from build123d import *

# Parameters (mm, degrees)
SKETCH1_R                      = 4.25
BOSS_EXTRUDE1_DEPTH            = 10
BOSS_EXTRUDE2_START            = -5
BOSS_EXTRUDE2_DEPTH            = 15
SKETCH3_W                      = 175
SKETCH3_H                      = 10
BOSS_EXTRUDE3_DEPTH            = 51.25
SKETCH4_W                      = 160
SKETCH4_H                      = 117.5
CUT_EXTRUDE1_DEPTH             = 10
CUT_EXTRUDE1_DIRECTION_2_REACH = 219.644
SKETCH5_W                      = 175
SKETCH5_H                      = 117.5
CUT_EXTRUDE2_DEPTH             = 15
SKETCH6_W                      = 5
SKETCH6_H                      = 15
BOSS_EXTRUDE4_DEPTH            = 3
CUT_EXTRUDE3_REACH             = 222.327
SKETCH7_W                      = 145
SKETCH7_H                      = 12.5


with BuildPart() as part:
    # Sketch1 → Boss-Extrude1 (new body)
    with BuildSketch(Plane(origin=(0, 0, 0), x_dir=(1, 0, 0), z_dir=(0, 1, 0))):
        Polygon((-87.5, 6.25), (87.5, 6.25), (87.5, -17), (75, -17), (75, -6.25), (-75, -6.25), (-75, -17), (-87.5, -17), align=None)
        with Locations(Location((-80, 0, 0), (0, 0, 270))):
            Circle(SKETCH1_R, mode=Mode.SUBTRACT)
        with Locations(Location((80, 0, 0), (0, 0, 270))):
            Circle(SKETCH1_R, mode=Mode.SUBTRACT)
    boss_extrude1 = extrude(amount=BOSS_EXTRUDE1_DEPTH)

    # Sketch2 → Boss-Extrude2 (add)
    with BuildSketch(Plane.XY.offset(17).offset(BOSS_EXTRUDE2_START)):
        Polygon((87.5, 130), (-87.5, 130), (-87.5, 0), (-75, 0), (-75, 105), (75, 105), (75, 0), (87.5, 0), align=None)
    boss_extrude2 = extrude(amount=BOSS_EXTRUDE2_DEPTH)

    # Sketch3 → Boss-Extrude3 (add)
    with BuildSketch(Plane.XY.offset(27)):
        with Locations((0, 110)):
            Rectangle(SKETCH3_W, SKETCH3_H)
    boss_extrude3 = extrude(amount=BOSS_EXTRUDE3_DEPTH)

    # Mirror2: Boss-Extrude1, Boss-Extrude2, Boss-Extrude3 across plane
    add(boss_extrude1.mirror(Plane.XY.offset(78.25)))
    add(boss_extrude2.mirror(Plane.XY.offset(78.25)))
    add(boss_extrude3.mirror(Plane.XY.offset(78.25)))

    # Sketch4 → Cut-Extrude1 (cut)
    with BuildSketch(Plane(origin=(0, 115, 0), x_dir=(1, 0, 0), z_dir=(0, 1, 0))):
        with Locations((0, -85.75)):
            Rectangle(SKETCH4_W, SKETCH4_H)
    extrude(amount=-CUT_EXTRUDE1_DEPTH, mode=Mode.SUBTRACT)

    # Cut-Extrude1 direction 2: up to this face of the body (flat: up to its plane)
    cut_extrude1_direction_2_end = Plane(part.part.faces().sort_by_distance((0, 130, 137))[0])
    # Sketch4 → Cut-Extrude1 direction 2 (cut, up to the picked face)
    with BuildSketch(Plane(origin=(0, 115, 0), x_dir=(1, 0, 0), z_dir=(0, 1, 0)), mode=Mode.PRIVATE) as cut_extrude1_direction_2_sk1:
        with Locations((0, -85.75)):
            Rectangle(SKETCH4_W, SKETCH4_H)
    cut_extrude1_direction_2_tool1 = split(extrude(cut_extrude1_direction_2_sk1.sketch, amount=CUT_EXTRUDE1_DIRECTION_2_REACH, mode=Mode.PRIVATE), bisect_by=cut_extrude1_direction_2_end, keep=Keep.BOTH, mode=Mode.PRIVATE)
    add(cut_extrude1_direction_2_tool1.solids().sort_by(Axis((0, 115, 85.75), (0, 1, 0)))[0], mode=Mode.SUBTRACT)

    # Sketch5 → Cut-Extrude2 (cut)
    with BuildSketch(Plane(origin=(0, 115, 0), x_dir=(1, 0, 0), z_dir=(0, 1, 0))):
        with Locations((0, -85.75)):
            Rectangle(SKETCH5_W, SKETCH5_H)
    extrude(amount=CUT_EXTRUDE2_DEPTH, mode=Mode.SUBTRACT)

    # Sketch6 → Boss-Extrude4 (add)
    with BuildSketch(Plane(origin=(0, 105, 0), x_dir=(1, 0, 0), z_dir=(0, 1, 0))):
        with Locations((-77.5, -137)):
            Rectangle(SKETCH6_W, SKETCH6_H)
        with Locations((77.5, -137)):
            Rectangle(SKETCH6_W, SKETCH6_H)
        Polygon((-80, -27), (-65, -27), (-80, -42), align=None)
        Polygon((80, -27), (65, -27), (80, -42), align=None)
    extrude(amount=BOSS_EXTRUDE4_DEPTH)

    # Sketch7 → Cut-Extrude3 (cut, up to next)
    with BuildSketch(Plane(origin=(0, 10, 0), x_dir=(1, 0, 0), z_dir=(0, 1, 0)), mode=Mode.PRIVATE) as cut_extrude3_sk1:
        with Locations((0, -156.5)):
            Rectangle(SKETCH7_W, SKETCH7_H)
    cut_extrude3_tool1 = extrude(cut_extrude3_sk1.sketch, amount=-CUT_EXTRUDE3_REACH, mode=Mode.PRIVATE) & part.part
    add(cut_extrude3_tool1.solids().sort_by_distance((0, 10, 156.5))[0], mode=Mode.SUBTRACT)


solid = part.part
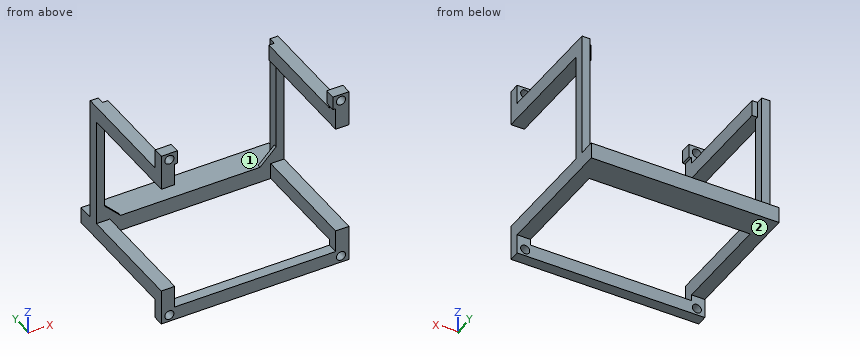
The model under review builds one solid part; all positions refer to its coordinate system, in mm. Face numbers are marked on the shaded views. Round coordinates to 2 decimals unless told otherwise and drop trailing zeros. Write each loop counter-clockwise with the first axis right and the second up, starting at its lowest first coordinate (ties: lowest second). Pieces come first, ordered by that corner, then holes. Notation, with made-up numbers: M 56,-32.5 L 70,-32.5 A32 cw 70,0.5 Z; hole C 6.25,-18.5 d10. An arc over 180 degrees is marked long. Answer as CSV lines item,"result". Start each with the question number.
Q1. Wall thickness on line 1 along X through (y, z) = (4.75, 156.5); line 2 along X through (y, z) = (3.25, 0); line 3 along X through (y, z) = (47, 138.5): over which ranges is each line inside the solid? List them lowest first.
Q2. Consider section D-D, the plane z = 61. Give the boundary of the cut face in (x, y), then the cut area to 3 significant figures.
Q3. Consider section A-A, the plane z = 0. Give the boundary of the cut face in (x, y).
Q4. Consider section B-B, the plane y = 33. Give the boundary of the cut face in (x, z).
Q5. Clearance check with flat-ended pins moving along their axes: P1, Ø16.5, axis at x = 78.5, z = 156.5, coming from the +Y side; P2, Ø10, axis at x = -81.5, y = 34, coming from the -Z side; P3, Ø5, axis at x = 13.5, y = 106.5, coming from the +Z side; P4, Ø11, axis at x = -80, z = 0, coming from the -Y side. State where each tip first meets the part, or that it passes through.
Q6. Consider section C-C, the plane x = -30. Give the boundary of the cut face in (y, z).
Q7. The part is to be moulded in two halves that separate along X. For the marked faces 1 and 2, say which applies: +X half, -X half, draft (parallel to the pull), parting line (faces both ways), or undercut.
Result set:
1,line 1,"x = -87.5 to -84.25, -75.75 to -72.5, 72.5 to 75.75, 84.25 to 87.5"
1,line 2,"x = -87.5 to -84.25, -75.75 to 75.75, 84.25 to 87.5"
1,line 3,"x = -87.5 to -75, 75 to 87.5"
2,outline,"M -87.5,105 L -80,105 L -80,115 L -87.5,115 Z; M 80,105 L 87.5,105 L 87.5,115 L 80,115 Z"
2,area,"150 mm²"
3,outline,"M -87.5,0 L -84.25,0 L -84.25,10 L -87.5,10 Z; M -75.75,0 L 75.75,0 L 75.75,10 L -75.75,10 Z; M 84.25,0 L 87.5,0 L 87.5,10 L 84.25,10 Z"
4,outline,"M -87.5,12 L -75,12 L -75,27 L -87.5,27 Z; M -87.5,129.5 L -75,129.5 L -75,144.5 L -87.5,144.5 Z; M 75,12 L 87.5,12 L 87.5,27 L 75,27 Z; M 75,129.5 L 87.5,129.5 L 87.5,144.5 L 75,144.5 Z"
5,P1,"stops at y = 10"
5,P2,"stops at z = 12"
5,P3,"stops at z = 27"
5,P4,"stops at y = 0"
6,outline,"M 0,-6.25 L 10,-6.25 L 10,6.25 L 0,6.25 Z; M 105,12 L 130,12 L 130,27 L 105,27 Z"
7,face 1,"undercut"
7,face 2,"draft"
